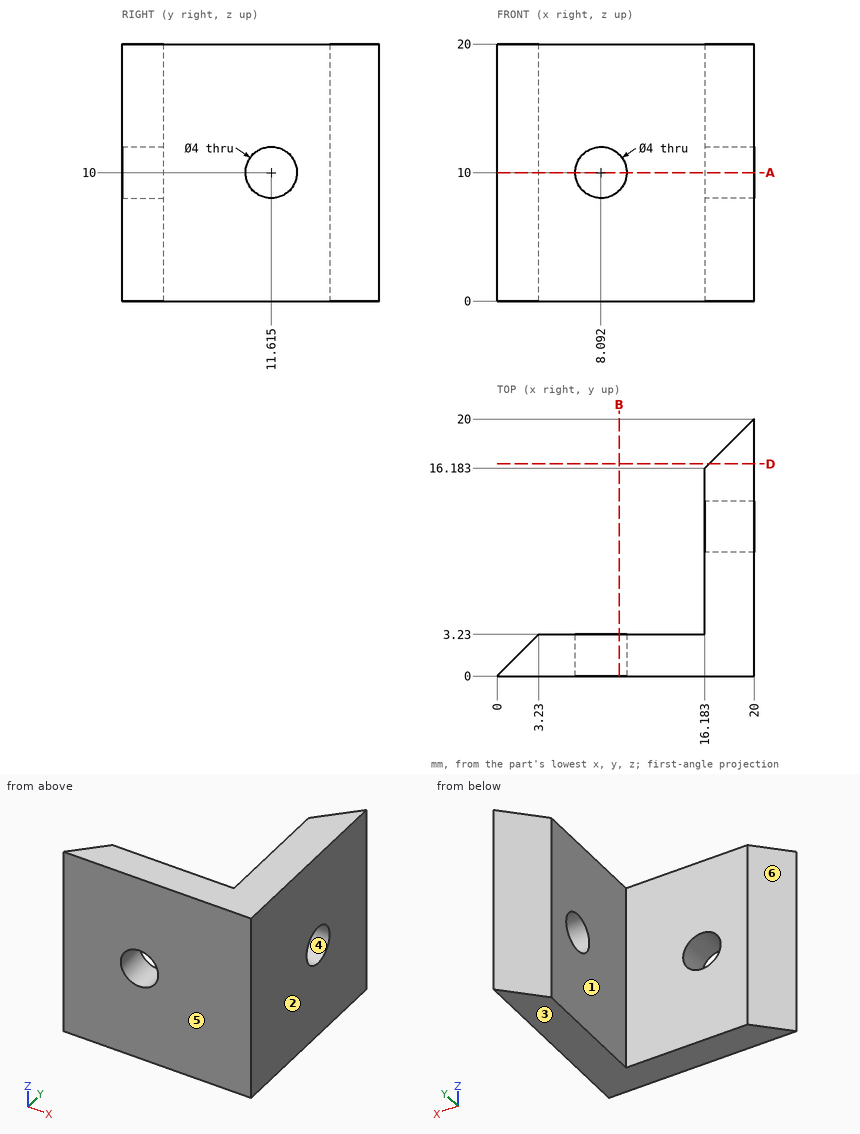
Verification items for this drawing (mm, ordinates from the low corner). A direction names the side the tool comes from. Give positions to 0.01 mm unless a question says otherwise; leave off trailing zeros. Write each loop counter-clockwise with the first axis right and the second up, starting at its lowest first coordinate (ties: lowest second). Pieces come first, ordered by that corner, then holes.
1) Gauge pin test, flat ends, axial feed: pin 1 (10.5 mm diameter, centred on x = 9, z = 6.5, fed in from +Y); pin 2 (6.5 mm diameter, centred on y = 12, z = 13.5, fed in from -X); pin 3 (10 mm diameter, centred on x = 13.5, z = 17.5, fed in from +Y). Record the tip position at first contact, or that the pin passes through.
2) Release check for a two-part mould opening along Y. For the marked faces 3, 4, 5 and 6 record: pulls with the +Y half, pulls with the -Y half, needs draft (parallel to the pull), parting line crosses it, or undercut.
3) Access from +Z, -Z, +X, -X, +Y, -Y to the whole of each face (thin tool, end or side, straight path). Record for the marked faces 1 and 2.
4) Section check D-D, the plane y = 16.5. Record the boundary of the cut face in (x, z), and give its area (3 significant figures).
5) Material ranges on L1, parallel to X at y = 7.5, z = 2.25; L2, parallel to Y at x = 15, z = 8.5; L3, parallel to X at y = 1.95, z = 10, recorded low to high.
6) Section check B-B, the plane x = 9.5. Record the boundary of the cut face in (y, z).
7) Section check A-A, the plane z = 10. Record the boundary of the cut face in (x, y) (1 decimal).
Computed:
1. pin 1: stops at y = 3.23
1. pin 2: stops at x = 16.18
1. pin 3: stops at y = 18.5
2. face 3: needs draft
2. face 4: undercut
2. face 5: pulls with the -Y half
2. face 6: pulls with the +Y half
3. face 1: +Z, -Z, -X, +Y
3. face 2: +Z, -Z, +X, +Y, -Y
4. outline: (16.5, 0) - (20, 0) - (20, 20) - (16.5, 20) - close
4. area: 70.0 mm2
5. L1: x = 16.18 to 20
5. L2: y = 0 to 3.23
5. L3: x = 1.95 to 6.09, 10.09 to 20
6. outline: (0, 0) - (3.23, 0) - (3.23, 8.58) - (0, 8.58) - close; (0, 11.42) - (3.23, 11.42) - (3.23, 20) - (0, 20) - close
7. outline: (0, 0) - (6.1, 0) - (6.1, 3.2) - (3.2, 3.2) - close; (10.1, 0) - (20, 0) - (20, 9.6) - (16.2, 9.6) - (16.2, 3.2) - (10.1, 3.2) - close; (16.2, 13.6) - (20, 13.6) - (20, 20) - (16.2, 16.2) - close
